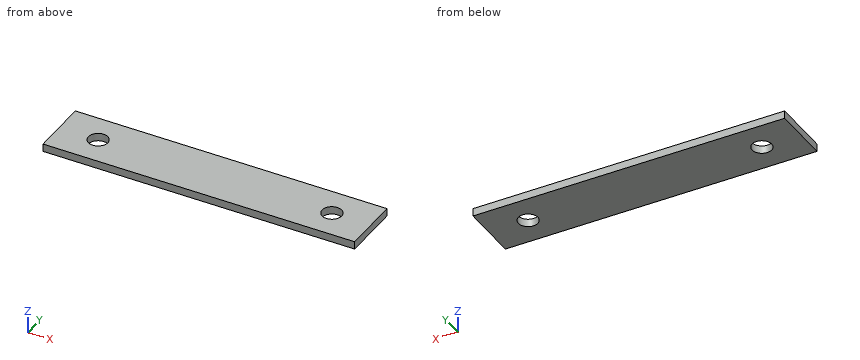
from build123d import *

# Parameters (mm, degrees)
SKETCH1_W          = 80
SKETCH1_H          = 15
BASE_FLANGE1_DEPTH = 2
CUT_EXTRUDE1_REACH = 83.419
SKETCH6_R          = 2.5


# Sheet-metal steps are written as plain solids
with BuildPart() as part:
    # Sketch1 → Base-Flange1 (new body)
    with BuildSketch(Plane.XY):
        with Locations((40, 7.5)):
            Rectangle(SKETCH1_W, SKETCH1_H)
    extrude(amount=-BASE_FLANGE1_DEPTH)

    # Sketch6 → Cut-Extrude1 (cut, up to next)
    with BuildSketch(Plane.XY, mode=Mode.PRIVATE) as cut_extrude1_sk1:
        with Locations((10, 7.5)):
            Circle(SKETCH6_R)
    cut_extrude1_tool1 = extrude(cut_extrude1_sk1.sketch, amount=-CUT_EXTRUDE1_REACH, mode=Mode.PRIVATE) & part.part
    # Sketch6 → Cut-Extrude1 (cut, up to next)
    with BuildSketch(Plane.XY, mode=Mode.PRIVATE) as cut_extrude1_sk2:
        with Locations((70, 7.5)):
            Circle(SKETCH6_R)
    cut_extrude1_tool2 = extrude(cut_extrude1_sk2.sketch, amount=-CUT_EXTRUDE1_REACH, mode=Mode.PRIVATE) & part.part
    add(cut_extrude1_tool1.solids().sort_by_distance((10, 7.5, 0))[0], mode=Mode.SUBTRACT)
    add(cut_extrude1_tool2.solids().sort_by_distance((70, 7.5, 0))[0], mode=Mode.SUBTRACT)


solid = part.part
The model under review builds one solid part; all positions refer to its coordinate system, in mm. Give positions to 0.01 mm unless a question says otherwise; leave off trailing zeros. Order: outer loops, then holes, each group sorted by start corner. A loop starts at its lowest first (then second) coordinate and runs counter-clockwise, first axis right, second up. Notation, with made-up numbers: M -31.75,71 L -11.75,71 A28 cw -11.75,93 Z; hole C -6.5,-19.5 d9. An arc over 180 degrees is marked long. One line per question, with ' | ' between items. Start each with the question number.
1) Consider section C-C, the plane z = -0.85. Give the boundary of the cut face in (x, y).
2) Wall thickness on L1, parallel to Y at x = 10, z = -1.5; L2, parallel to X at y = 9, z = -0.3; L3, parallel to X at y = 9.5, z = -1.8: over which ranges is each line inside the solid? List them lowest first. Write a range as from..to.
3) Consider section B-B, the plane y = 7.5. Give the boundary of the cut face in (x, z), then the cut area to 3 significant figures.
4) Clearance check with a flat-ended pin moving along its axis: P1, Ø3, axis at x = 10, y = 7.5, coming from the -Z side. State where the tip first meets the part, or that it passes through.
5) Consider section A-A, the plane x = 71.5. Give the boundary of the cut face in (y, z).
Found:
1) outline: M 0,0 L 80,0 L 80,15 L 0,15 Z; hole C 10,7.5 d5; hole C 70,7.5 d5
2) L1: y = 0..5, 10..15 | L2: x = 0..8, 12..68, 72..80 | L3: x = 0..8.5, 11.5..68.5, 71.5..80
3) outline: M 0,-2 L 7.5,-2 L 7.5,0 L 0,0 Z; M 12.5,-2 L 67.5,-2 L 67.5,0 L 12.5,0 Z; M 72.5,-2 L 80,-2 L 80,0 L 72.5,0 Z | area: 140 mm²
4) P1: passes through
5) outline: M 0,-2 L 5.5,-2 L 5.5,0 L 0,0 Z; M 9.5,-2 L 15,-2 L 15,0 L 9.5,0 Z
